```python
from build123d import *

# Parameters (mm, degrees)
PCB_DIMENSIONS_W    = 47.716732244
PCB_DIMENSIONS_H    = 77.636732244
BOSS_EXTRUDE3_DEPTH = 1.5
SKETCH5_W           = 47.716732244
SKETCH5_H           = 77.636732244
SKETCH5_W_2         = 43.474091557
SKETCH5_H_2         = 73.394091557
BOSS_EXTRUDE5_DEPTH = 30
FILLET1_R           = 1
SKETCH9_W           = 1.93805105
SKETCH9_H           = 42
SKETCH9_W_2         = 1.938051049
BOSS_EXTRUDE6_DEPTH = 5
SKETCH14_W          = 15
SKETCH14_H          = 2.5
BOSS_EXTRUDE7_DEPTH = 3
SKETCH15_W          = 75.636732244
SKETCH15_H          = 3
BOSS_EXTRUDE8_DEPTH = 46
SKETCH17_W          = 39.522771214
SKETCH17_H          = 62.982276128
CUT_EXTRUDE1_DEPTH  = 3
CUT_EXTRUDE2_DEPTH  = 3
SKETCH19_W          = 11
SKETCH19_H          = 5
CUT_EXTRUDE3_DEPTH  = 10
FILLET2_R           = 1
SCALE1_SCALE        = 0.99


with BuildPart() as part:
    # PCB Dimensions → Boss-Extrude3 (new body)
    with BuildSketch(Plane(origin=(0, 0, 0), x_dir=(1, 0, 0), z_dir=(0, 1, 0))):
        with Locations((20.322832216, -35.282832216)):
            Rectangle(PCB_DIMENSIONS_W, PCB_DIMENSIONS_H)
    extrude(amount=BOSS_EXTRUDE3_DEPTH)

    # Sketch5 → Boss-Extrude5 (add)
    with BuildSketch(Plane(origin=(0, 1.5, 0), x_dir=(1, 0, 0), z_dir=(0, 1, 0))):
        with Locations((20.322832216, -35.282832216)):
            Rectangle(SKETCH5_W, SKETCH5_H)
        with Locations((20.322832217, -35.282832217)):
            Rectangle(SKETCH5_W_2, SKETCH5_H_2, mode=Mode.SUBTRACT)
    extrude(amount=BOSS_EXTRUDE5_DEPTH)

    # Fillet1
    fillet1_edges = [part.edges().sort_by_distance(p)[0] for p in [
        (42.059877995, 16.5, -1.414213562),
        (-1.414213562, 16.5, -1.414213562),
        (-1.414213562, 16.5, 71.979877995),
        (42.059877995, 16.5, 71.979877995),
        (44.181198338, 15.75, 74.101198338),
        (-3.535533906, 15.75, 74.101198338),
        (-3.535533906, 15.75, -3.535533906),
        (44.181198338, 15.75, -3.535533906),
    ]]
    fillet(fillet1_edges, radius=FILLET1_R)

    # Sketch9 → Boss-Extrude6 (add)
    with BuildSketch(Plane(origin=(0, 1.5, 0), x_dir=(1, 0, 0), z_dir=(0, 1, 0))):
        with Locations((-0.88911969, -49.979881394)):
            Rectangle(SKETCH9_W, SKETCH9_H)
        with Locations((41.534784122, -49.979881394)):
            Rectangle(SKETCH9_W_2, SKETCH9_H)
    extrude(amount=BOSS_EXTRUDE6_DEPTH)

    # Sketch14 → Boss-Extrude7 (add)
    with BuildSketch(Plane(origin=(0, 1.5, 0), x_dir=(1, 0, 0), z_dir=(0, 1, 0))):
        with Locations((6.085786438, -26.529881394)):
            Rectangle(SKETCH14_W, SKETCH14_H)
        with Locations((34.559877995, -26.529881394)):
            Rectangle(SKETCH14_W, SKETCH14_H)
    extrude(amount=BOSS_EXTRUDE7_DEPTH)

    # Sketch15 → Boss-Extrude8 (add)
    with BuildSketch(Plane(origin=(44.181198338, 0, 0), x_dir=(0, 0, -1), z_dir=(1, 0, 0))):
        with Locations((-35.282832216, 15.5)):
            Rectangle(SKETCH15_W, SKETCH15_H)
    extrude(amount=-BOSS_EXTRUDE8_DEPTH)

    # Sketch17 → Cut-Extrude1 (cut)
    with BuildSketch(Plane(origin=(0, 17, 0), x_dir=(1, 0, 0), z_dir=(0, 1, 0))):
        with Locations((20.322832216, -32.052584673)):
            Rectangle(SKETCH17_W, SKETCH17_H)
    extrude(amount=-CUT_EXTRUDE1_DEPTH, mode=Mode.SUBTRACT)

    # Sketch18 → Cut-Extrude2 (cut)
    with BuildSketch(Plane(origin=(0, 17, 0), x_dir=(1, 0, 0), z_dir=(0, 1, 0))):
        with BuildLine():
            Line((-1.414213562, -9.585786438), (28.585786438, -9.585786438))
            Line((28.585786438, -9.585786438), (28.585786438, 1.414213562))
            Line((28.585786438, 1.414213562), (-0.414213562, 1.414213562))
            ThreePointArc((-0.414213562, 1.414213562), (-1.121320344, 1.121320344), (-1.414213562, 0.414213562))
            Line((-1.414213562, 0.414213562), (-1.414213562, -9.585786438))
        make_face()
    extrude(amount=-CUT_EXTRUDE2_DEPTH, mode=Mode.SUBTRACT)

    # Sketch19 → Cut-Extrude3 (cut)
    with BuildSketch(Plane(origin=(44.181198338, 0, 0), x_dir=(0, 0, -1), z_dir=(1, 0, 0))):
        with Locations((-5.464466094, 21.15)):
            Rectangle(SKETCH19_W, SKETCH19_H)
    extrude(amount=-CUT_EXTRUDE3_DEPTH, mode=Mode.SUBTRACT)

    # Fillet2
    fillet2_edges = [part.edges().sort_by_distance(p)[0] for p in [
        (43.120538167, 23.65, -0.035533906),
        (43.120538167, 18.65, -0.035533906),
        (43.120538167, 18.65, 10.964466094),
        (43.120538167, 23.65, 10.964466094),
    ]]
    fillet(fillet2_edges, radius=FILLET2_R)


with BuildPart() as part_1:
    # Scale1: scaled about (20.30907108, 12.22563111, 37.095530551)
    add(part.part.scale(SCALE1_SCALE).moved(Location((0.203090711, 0.122256311, 0.370955306))))


solid = part_1.part
```
Here's how the part is built. I have some questions about the finished solid (model axes, mm). A direction names the side the tool comes from. Coordinates: 2 decimals unless noted, no trailing zeros. Loops run counter-clockwise (first coordinate to the right, second up) from the corner with the lowest first, then second, coordinate; pieces in that order, holes last. Notation, with made-up numbers: (60, 74.5) - (97, 74.5) arc R31 cw to (97, 105.5) - close; hole circle Ø10 at (-17, 60). An arc over 180 degrees is marked (long way). Return JSON: item names as keys, results as strings. Group by question number.
Item 1: If we section it at B-B on x = 38: Write out the boundary of the cut face in (y, z), and give its area (3 significant figures).
Item 2: If we section it at D-D on y = 21: Write out the boundary of the cut face in (x, z).
Item 3: Will these pins go through, and if not, where does the flat tip stop? P1, Ø21.5, axis at x = 25, z = 19.5, coming from the +Y side; P2, Ø8, axis at x = 29, z = 63.5, coming from the +Y side; P3, Ø2, axis at x = 17.5, z = 48.5, coming from the +Y side.
Item 4: We'd pull the mould along X, two halves only. Please class faces 6 (the face through (0, 4, 29.061)), 7 (the face through (43, 21, 11.226)), 8 (the face through (43.942, 16, 36)): +X half, -X half, draft (parallel to the pull), parting line (faces both ways), or undercut.
Item 5: I need wall thicknesses on line 1 (X direction, y = 18.5, z = 22); line 2 (Z direction, x = 20, y = 3); line 3 (Y direction, x = -1, z = 12.5). Which ranges of each line are inside material? Lowest first, please. Write a range as from..to.
Item 6: If we section it at C-C on z = 23: Write out the boundary of the cut face in (x, y), and give its area (3 significant figures).
Item 7: On a 3-axis mill with a long thin cutter (end or side, diameter ignored), from which of +Z, -Z, +X, -X, +Y, -Y can I reach the whole of each face in a straight line? I mean faces 1 (the face through (13.653, 3, 27)), 2 (the face through (20, 15, -3.129)), 3 (the face through (-3.297, 15, 36)), 4 (the face through (43, 23.536, 6)), 5 (the face through (20, 16, -1.029)). Say none if no direction works.
Calculated:
{
 "1": {"outline": "(0.12, -3.13) - (31.31, -3.13) - (31.31, -1.03) - (16.95, -1.03) - (16.95, 0.93) - (13.98, 0.93) - (13.98, -1.03) - (1.61, -1.03) - (1.61, 25.4) - (4.58, 25.4) - (4.58, 27.87) - (1.61, 27.87) - (1.61, 71.63) - (13.98, 71.63) - (13.98, 63.28) - (16.95, 63.28) - (16.95, 71.63) - (31.31, 71.63) - (31.31, 73.73) - (0.12, 73.73) - close", "area": "277 mm^2"},
 "2": {"outline": "(-3.3, -2.14) arc R0.99 ccw to (-2.31, -3.13) - (42.95, -3.13) arc R0.99 ccw to (43.94, -2.14) - (43.94, 0.34) - (41.84, 0.34) - (41.84, -0.04) arc R0.99 cw to (40.85, -1.03) - (-0.21, -1.03) arc R0.99 cw to (-1.2, -0.04) - (-1.2, 70.64) arc R0.99 cw to (-0.21, 71.63) - (40.85, 71.63) arc R0.99 cw to (41.84, 70.64) - (41.84, 11.23) - (43.94, 11.23) - (43.94, 72.74) arc R0.99 ccw to (42.95, 73.73) - (-2.31, 73.73) arc R0.99 ccw to (-3.3, 72.74) - close"},
 "3": {"P1": "stops at y = 4.58", "P2": "stops at y = 16.95", "P3": "stops at y = 1.61"},
 "4": {"face 6": "undercut", "face 7": "draft", "face 8": "+X half"},
 "5": {"line 1": "x = -3.3..-1.2, 41.84..43.94", "line 2": "z = -3.13..-1.03, 71.63..73.73", "line 3": "y = 0.12..1.61, 13.98..16.95"},
 "6": {"outline": "(-3.3, 0.12) - (43.94, 0.12) - (43.94, 31.31) - (41.84, 31.31) - (41.84, 16.95) - (39.89, 16.95) - (39.89, 13.98) - (41.84, 13.98) - (41.84, 1.61) - (-1.2, 1.61) - (-1.2, 13.98) - (0.76, 13.98) - (0.76, 16.95) - (-1.2, 16.95) - (-1.2, 31.31) - (-3.3, 31.31) - close", "area": "207 mm^2"},
 "7": {"face 1": "+Y", "face 2": "-Z, +X, -X, +Y, -Y", "face 3": "+Z, -Z, -X, +Y, -Y", "face 4": "+X", "face 5": "none"}
}
